```python
from build123d import *

# Parameters (mm, degrees)
BOSS_EXTRUDE1_DEPTH = 10
SKETCH2_OUTSIDE_W   = 88.614
SKETCH2_OUTSIDE_H   = 38.614
CUT_EXTRUDE1_DEPTH  = 55.083269132
SKETCH3_R           = 13
BOSS_EXTRUDE2_DEPTH = 150
SKETCH15_R          = 12.5
CUT_EXTRUDE2_DEPTH  = 154.495928285


with BuildPart() as part:
    # Sketch1 → Boss-Extrude1 (new, symmetric)
    with BuildSketch(Plane(origin=(0, 0, 0), x_dir=(1, 0, 0), z_dir=(0, 1, 0))):
        with BuildLine():
            Line((4.442128661, 20), (-29, 20))
            ThreePointArc((-29, 20), (-33.242640687, 18.242640687), (-35, 14))
            Line((-35, 14), (-35, -14))
            ThreePointArc((-35, -14), (-33.242640687, -18.242640687), (-29, -20))
            Line((-29, -20), (4.442128661, -20))
            ThreePointArc((4.442128661, -20), (9.877208627, -19.42557582), (15.072131567, -17.727685058))
            Line((15.072131567, -17.727685058), (30.270770125, -10.918694984))
            ThreePointArc((30.270770125, -10.918694984), (33.714393532, -7.967227328), (35, -3.617868812))
            Line((35, -3.617868812), (35, 3.617868812))
            ThreePointArc((35, 3.617868812), (33.714393532, 7.967227328), (30.270770125, 10.918694984))
            Line((30.270770125, 10.918694984), (15.072131567, 17.727685058))
            ThreePointArc((15.072131567, 17.727685058), (9.877208627, 19.42557582), (4.442128661, 20))
        make_face()
    boss_extrude1 = extrude(amount=BOSS_EXTRUDE1_DEPTH, both=True)

    # Sketch2 outside → Cut-Extrude1 (cut, through all)
    with BuildSketch(Plane.XY.offset(20)):
        Rectangle(SKETCH2_OUTSIDE_W, SKETCH2_OUTSIDE_H)
        with BuildLine():
            Line((-35, 10), (-23.9, 10))
            ThreePointArc((-23.9, 10), (-12.33766892, 2.25), (-0.77533784, 10))
            Line((-0.77533784, 10), (35, 10))
            Line((35, 10), (35, 6))
            Line((35, 6), (1.651165913, 6))
            ThreePointArc((1.651165913, 6), (-12.33766892, -1.75), (-26.326503754, 6))
            Line((-26.326503754, 6), (-35, 6))
            Line((-35, 6), (-35, 10))
        make_face(mode=Mode.SUBTRACT)
    extrude(amount=-CUT_EXTRUDE1_DEPTH, mode=Mode.SUBTRACT)

    # Sketch3 → Boss-Extrude2 (add)
    with BuildSketch(Plane.XZ.offset(-6)):
        with Locations(Location((20, 0, 0), (0, 0, 270))):
            Circle(SKETCH3_R)
    extrude(amount=BOSS_EXTRUDE2_DEPTH)

    # Mirror1: Boss-Extrude1 across plane
    add(boss_extrude1.mirror(Plane.ZX.offset(10)))

    # Sketch15 → Cut-Extrude2 (cut, through all)
    with BuildSketch(Plane.XY.offset(20)):
        with Locations((-12.33766892, 14.75)):
            Circle(SKETCH15_R)
    extrude(amount=-CUT_EXTRUDE2_DEPTH, mode=Mode.SUBTRACT)


solid = part.part
```
For this review, take the finished solid that the model builds, in its own axes (mm). A direction names the side the tool comes from. Round coordinates to 2 decimals unless told otherwise and drop trailing zeros. Write each loop counter-clockwise with the first axis right and the second up, starting at its lowest first coordinate (ties: lowest second). Pieces come first, ordered by that corner, then holes. Notation, with made-up numbers: M 12.25,39.5 L 71.25,39.5 A16 cw 71.25,48.5 Z; hole C -0.75,-30.75 d10. An arc over 180 degrees is marked long. One line per item, written item: value. Start each with the question number.
(1) We need section A-A (z = 0). Give the boundary of the cut face in (x, y), and give its area (3 significant figures).
(2) Wall thickness on line 1 (X direction, y = 14.75, z = -1); line 2 (Y direction, x = -13, z = 16.5); line 3 (X direction, y = 14.75, z = 7): over which ranges is each line inside the solid? List them lowest first.
(3) We need section B-B (y = 14.75). Give the boundary of the cut face in (x, z).
(4) Insertion check: pin 1 (7 mm diameter, centred on x = -29, z = -7.5, fed in from -Y); pin 2 (15 mm diameter, centred on x = -12.34, y = 14.75, fed in from +Z); pin 3 (2 mm diameter, centred on y = -81.5, z = 10, fed in from +X); pin 4 (2 mm diameter, centred on y = -45.5, z = 4, fed in from +X). Each pin has a flat end and moves straight along its axis. Give the tip position at first contact, or say it passes through.
(5) We need section C-C (x = -4.5). Give the boundary of the cut face in (y, z).
(6) Machinability: for faces 1 (the flat face through (-12, 28, -20)), 2 (the cylindrical face through (32.89, -67.95, 1.69)), which of the approach directions +Z, -Z, +X, -X, +Y, -Y give a long, thin tool a straight path to every point of the face, cutting with its end or side? Answer none if there is none.
(7) We need section D-D (x = 20). Give the boundary of the cut face in (y, z), and give its area (3 significant figures).
(8) The part is to be moulded in two halves that separate along X. For faces 3 (the flat face through (22.57, 17.83, 14.37)), 4 (the flat face through (7, 6, -4)), 5 (the flat face through (-31, 6, 0)), say which applies: released by +X, released by -X, zero draft, split by the parting line, or undercut.
Result:
1. outline: M -35,6 L -26.33,6 A16.5 ccw 1.65,6 L 7,6 L 7,-144 L 33,-144 L 33,6 L 35,6 L 35,30 L -35,30 Z; hole C -12.34,14.75 d25
1. area: 5,240 mm²
2. line 1: -35 to -24.84, 0.16 to 35
2. line 2: -1.74 to 2.27, 27.23 to 30
2. line 3: -35 to -24.84, 0.16 to 34.25
3. outline: M -35,-14 A6 ccw -29,-20 L -24.84,-20 L -24.84,20 L -29,20 A6 ccw -35,14 Z; M 0.16,-20 L 4.44,-20 A26 ccw 15.07,-17.73 L 30.27,-10.92 A8 ccw 35,-3.62 L 35,3.62 A8 ccw 30.27,10.92 L 15.07,17.73 A26 ccw 4.44,20 L 0.16,20 Z
4. pin 1: y = 4.8
4. pin 2: through
4. pin 3: x = 29.38
4. pin 4: x = 32.65
5. outline: M 0.23,-20 L 5.01,-20 L 5.01,20 L 0.23,20 Z; M 24.49,-20 L 30,-20 L 30,20 L 24.49,20 Z
6. face 1: -Z, +X, -X, +Y, -Y
6. face 2: -Y
7. outline: M -144,-13 L 6,-13 L 6,-15.52 L 30,-15.52 L 30,15.52 L 6,15.52 L 6,13 L -144,13 Z
7. area: 4,640 mm²
8. face 3: released by +X
8. face 4: undercut
8. face 5: zero draft
